For this review, take the finished solid that the model builds, in its own axes (mm). A direction names the side the tool comes from. Give positions to 0.01 mm unless a question says otherwise; leave off trailing zeros. Loops run counter-clockwise (first coordinate to the right, second up) from the corner with the lowest first, then second, coordinate; pieces in that order, holes last. Notation, with made-up numbers: (-2.75, -5) -> (6.25, -5) arc R12 ccw to (6.25, 15) -> close; hole circle Ø8 at (60.5, 51.25). An arc over 180 degrees is marked (long way). One line per question, with ' | ' between items. Start each with the question number.
(1) Consider section C-C (y = -8.5). Write out the cut boundary in (x, z), and give its area (3 significant figures).
(2) Consider section D-D (y = -17.5). Write out the cut boundary in (x, z).
(3) Consider section B-B (x = 3). Write out the cut boundary in (y, z).
(4) Tool access review of faces 1 (the flat face through (-15, -13.252, 4)), 2 (the flat face through (13.252, 15, 4)), 3 (the flat face through (21.142, 15, 4)): name each direction out of +Z, -Z, +X, -X, +Y, -Y from which nothing blocks a thin tool from reaching the whole face with its end or side.
(5) Draft analysis for pull direction Y (two halves, no side actions). For faces 4 (the flat face through (13, 22.788, 6)), 5 (the flat face through (17, 16.138, 5)), 6 (the flat face through (-14.838, -17, 5)), 7 (the flat face through (-4, -24.252, 1)), state which applies: +Y half, -Y half, draft (parallel to the pull), parting line (faces both ways), or undercut.
(6) Consider section A-A (z = 4.25). Write out the cut boundary in (x, y).
(7) Insertion check: P1, Ø23.5, axis at x = 9, y = -10, coming from the +Z side; P2, Ø1.4, axis at y = 15.5, z = 4.5, coming from the +X side; P3, Ø1, axis at x = -15.5, z = 5, coming from the -Y side. Each pin has a flat end and moves straight along its axis. Give the tip position at first contact, or say it passes through.
(8) Wall thickness on probe 1 along Y at (x, z) = (20.5, 7.25); probe 2 along X at (y, z) = (-14, 6); probe 3 along Z at (x, y) = (10.5, -7.5): over which ranges is each line inside the solid? List them lowest first.
from build123d import *

# Parameters (mm, degrees)
F0_R     = 6.5
F1_DEPTH = 1.85
F3_DEPTH = 8
F4_W     = 1.3
F4_H     = 7.89
F4_W_2   = 7.89
F4_H_2   = 1.3
F5_DEPTH = 6
F6_R     = 1


with BuildPart() as f1:
    # F0 (on Top) → F1 (new body)
    with BuildSketch(Plane.XY):
        with BuildLine():
            Line((-24.288, -24.252), (24.252, -24.252))
            Line((24.252, -24.252), (24.252, 24.288))
            Line((24.252, 24.288), (1.712, 24.288))
            ThreePointArc((1.712, 24.288), (-16.672776, 16.672776), (-24.288, -1.712))
            Line((-24.288, -1.712), (-24.288, -24.252))
        make_face()
        with Locations((-5.005514, 5.005514)):
            Circle(F0_R, mode=Mode.SUBTRACT)
    extrude(amount=F1_DEPTH)

    # F2 (on face) → F3 (join)
    with BuildSketch(Plane.XY.offset(1.85)):
        with BuildLine():
            Line((-24.288, -1.712), (-24.288, -24.252))
            Line((-24.288, -24.252), (-22.788, -24.252))
            Line((-22.788, -24.252), (-22.788, -1.712))
            ThreePointArc((-22.788, -1.712), (-15.612116, 15.612116), (1.712, 22.788))
            Line((1.712, 22.788), (24.252, 22.788))
            Line((24.252, 22.788), (24.252, 24.288))
            Line((24.252, 24.288), (1.712, 24.288))
            ThreePointArc((1.712, 24.288), (-16.672776, 16.672776), (-24.288, -1.712))
        make_face()
    extrude(amount=F3_DEPTH)

    # F4 (on face) → F5 (join)
    with BuildSketch(Plane.XY.offset(1.85)):
        with Locations((-15.488, -17.197)):
            Rectangle(F4_W, F4_H)
        with Locations((17.197, 15.488)):
            Rectangle(F4_W_2, F4_H_2)
    extrude(amount=F5_DEPTH)

    # F6
    f6_edges = [f1.edges().sort_by_distance(p)[0] for p in [
        (-23.538, -24.252, 9.85),
        (24.252, 23.538, 9.85),
        (-24.288, -12.982, 0),
        (-15.488, -21.142, 7.85),
        (-15.488, -13.252, 7.85),
        (13.252, 15.488, 7.85),
        (21.142, 15.488, 7.85),
        (24.252, -24.252, 0.925),
    ]]
    fillet(f6_edges, radius=F6_R)


solid = f1.part
A:
1) outline: (-24.29, 1) arc R1 ccw to (-23.29, 0) -> (24.25, 0) -> (24.25, 1.85) -> (-22.79, 1.85) -> (-22.79, 9.85) -> (-24.29, 9.85) -> close | area: 102 mm^2
2) outline: (-24.29, 1) arc R1 ccw to (-23.29, 0) -> (24.25, 0) -> (24.25, 1.85) -> (-14.84, 1.85) -> (-14.84, 7.85) -> (-16.14, 7.85) -> (-16.14, 1.85) -> (-22.79, 1.85) -> (-22.79, 9.85) -> (-24.29, 9.85) -> close
3) outline: (-24.25, 0) -> (23.29, 0) arc R1 ccw to (24.29, 1) -> (24.29, 9.85) -> (22.79, 9.85) -> (22.79, 1.85) -> (-24.25, 1.85) -> close
4) face 1: +Z, +X | face 2: +Z, -Y | face 3: +Z, +X, -Y
5) face 4: undercut | face 5: undercut | face 6: draft | face 7: -Y half
6) outline: (-24.29, -24.25) -> (-22.79, -24.25) -> (-22.79, -1.71) arc R24.5 cw to (1.71, 22.79) -> (24.25, 22.79) -> (24.25, 24.29) -> (1.71, 24.29) arc R26 ccw to (-24.29, -1.71) -> close; (-16.14, -21.14) -> (-14.84, -21.14) -> (-14.84, -13.25) -> (-16.14, -13.25) -> close; (13.25, 14.84) -> (21.14, 14.84) -> (21.14, 16.14) -> (13.25, 16.14) -> close
7) P1: stops at z = 1.85 | P2: stops at x = 21.14 | P3: stops at y = -21.14
8) probe 1: y = 14.84 to 16.14, 22.79 to 24.29 | probe 2: x = -24.29 to -22.79, -16.14 to -14.84 | probe 3: z = 0 to 1.85
